from build123d import *

# Parameters (mm, degrees)
F0_W      = 76.2
F0_H      = 76.2
F1_DEPTH  = 76.2
F2_R      = 12.7
F4_DEPTH  = 12.7
F6_DEPTH  = 12.7
F7_W      = 25.4
F7_H      = 25.4
F8_DEPTH  = 25.4
F9_W      = 25.4
F9_H      = 25.4
F10_DEPTH = 25.4
F11_W     = 3.6200266331
F11_H     = 25.4
F12_DEPTH = 12.7
F13_W     = 5.1714666188
F13_H     = 16.2901245058
F13_R     = 2.3271590471
F14_DEPTH = 12.7
F16_DEPTH = 12.7


with BuildPart() as f1:
    # F0 (on Front) → F1 (new body)
    with BuildSketch(Plane.XZ):
        with Locations((38.1, 38.1)):
            Rectangle(F0_W, F0_H)
    extrude(amount=F1_DEPTH)

    # F2
    f2_edges = [f1.edges().sort_by_distance(p)[0] for p in [
        (38.1, -76.2, 76.2),
        (76.2, -38.1, 76.2),
        (38.1, 0, 76.2),
        (0, -38.1, 76.2),
        (76.2, -76.2, 38.1),
        (76.2, 0, 38.1),
        (0, -76.2, 38.1),
        (0, 0, 38.1),
        (0, -38.1, 0),
        (38.1, 0, 0),
        (76.2, -38.1, 0),
        (38.1, -76.2, 0),
    ]]
    fillet(f2_edges, radius=F2_R)

    # F3 (on face) → F4 (cut)
    with BuildSketch(Plane.XZ.offset(76.2)):
        with BuildLine():
            Line((15.24, 47.6933766934), (15.24, 38.1))
            ThreePointArc((15.24, 38.1), (21.992776406, 42.8966883467), (15.24, 47.6933766934))
        make_face()
        Polygon((27.94, 50.8), (27.94, 25.4), (40.64, 25.4), (40.64, 30.5915938972), (34.1505076285, 30.5915938972), (34.1505076285, 35.7831877943), (39.3421015257, 35.7831877943), (39.3421015257, 40.9747816915), (34.1505076285, 40.9747816915), (34.1505076285, 46.1663755887), (40.64, 46.1663755887), (40.64, 50.8), align=None)
        with BuildLine():
            ThreePointArc((45.72, 25.4), (58.42, 38.1), (45.72, 50.8))
            Line((45.72, 50.8), (45.72, 25.4))
        make_face()
    extrude(amount=-F4_DEPTH, mode=Mode.SUBTRACT)

    # F5 (on face) → F6 (cut)
    with BuildSketch(Plane.XZ.offset(76.2)):
        Polygon((23.7294812034, 22.97295762), (15.8522693162, 35.67295762), (15.8522693162, 22.97295762), (18.3922693162, 22.97295762), (18.3922693162, 25.51295762), (21.1894812034, 25.51295762), (21.1894812034, 22.97295762), align=None)
    extrude(amount=-F6_DEPTH, mode=Mode.SUBTRACT)

    # F7 (on face) → F8 (cut)
    with BuildSketch(Plane(origin=(0, 0, 0), x_dir=(1, 0, 0), z_dir=(0, 0, -1))):
        with Locations((38.1038359793, 38.1)):
            Rectangle(F7_W, F7_H)
    extrude(amount=-F8_DEPTH, mode=Mode.SUBTRACT)

    # F9 (on face) → F10 (join)
    with BuildSketch(Plane.XY.offset(76.2)):
        with Locations((38.1, -38.0961640207)):
            Rectangle(F9_W, F9_H)
    extrude(amount=F10_DEPTH)

    # F11 (on face) → F12 (cut)
    with BuildSketch(Plane(origin=(0, 0, 0), x_dir=(0, -1, 0), z_dir=(-1, 0, 0))):
        with BuildLine():
            ThreePointArc((16.548698768, 44.5045307279), (20.8982916063, 50.9688649327), (16.548698768, 57.4331991374))
            Line((16.548698768, 57.4331991374), (16.548698768, 44.5045307279))
        make_face()
        with BuildLine():
            ThreePointArc((16.548698768, 20.9743473679), (23.013450923, 29.5072691515), (16.548698768, 38.0401909351))
            Line((16.548698768, 38.0401909351), (16.548698768, 20.9743473679))
        make_face()
        with Locations((27.4087795988, 32.1229073822)):
            Rectangle(F11_W, F11_H)
        with BuildLine():
            Line((36.9759984314, 37.5230461359), (31.0288090259, 37.5230461359))
            ThreePointArc((31.0288090259, 37.5230461359), (39.5617289469, 24.9625075374), (48.0946488678, 37.5230461359))
            Line((48.0946488678, 37.5230461359), (42.1474650502, 37.5230461359))
            ThreePointArc((42.1474650502, 37.5230461359), (39.5617317408, 29.699298714), (36.9759984314, 37.5230461359))
        make_face()
        Polygon((51.9732572138, 54.6391973982), (51.9732572138, 29.2391973982), (59.5346949809, 30.1820965947), (59.5346949809, 35.2620965947), (53.9881583642, 35.2620965947), (53.9881583642, 40.3420965947), (59.0681583642, 40.3420965947), (59.0681583642, 45.4220965947), (53.9881583642, 45.4220965947), (53.9881583642, 50.5020965947), (58.9798856309, 49.5591973982), (58.9798856309, 54.6391973982), align=None)
    extrude(amount=-F12_DEPTH, mode=Mode.SUBTRACT)

    # F13 (on face) → F14 (cut)
    with BuildSketch(Plane(origin=(0, 0, 0), x_dir=(-1, 0, 0), z_dir=(0, 1, 0))):
        with BuildLine():
            ThreePointArc((-52.724421297, 37.3828077149), (-48.797749492, 44.5476863023), (-56.9577540953, 44.958248733))
            Line((-56.9577540953, 44.958248733), (-56.9577540953, 19.558248733))
            Line((-56.9577540953, 19.558248733), (-52.724421297, 19.558248733))
            Line((-52.724421297, 19.558248733), (-52.724421297, 37.3828077149))
        make_face()
        with Locations((-42.6646117121, 28.6022629589)):
            Rectangle(F13_W, F13_H)
        with BuildLine():
            Line((-37.4931432307, 36.7473252118), (-37.4931432307, 20.7157749683))
            Line((-37.4931432307, 20.7157749683), (-34.9074080586, 20.7157749683))
            Line((-34.9074080586, 20.7157749683), (-34.9074080586, 28.2144043595))
            ThreePointArc((-34.9074080586, 28.2144043595), (-31.9338152185, 31.1879971996), (-28.9602223784, 28.2144043595))
            Line((-28.9602223784, 28.2144043595), (-28.9602223784, 21.2329216301))
            Line((-28.9602223784, 21.2329216301), (-26.4202223784, 21.2329216301))
            Line((-26.4202223784, 21.2329216301), (-27.4545157021, 32.0930033922))
            ThreePointArc((-27.4545157021, 32.0930033922), (-30.6866828045, 35.3251704946), (-33.9188499069, 32.0930033922))
            Line((-33.9188499069, 32.0930033922), (-33.9188499069, 36.7473252118))
            Line((-33.9188499069, 36.7473252118), (-37.4931432307, 36.7473252118))
        make_face()
        Polygon((-23.4643667936, 45.8856336772), (-23.4643667936, 21.2329216301), (-21.2937723845, 21.1951211095), (-21.2937723845, 28.6565385759), (-18.9875140786, 21.1951211095), (-15.4602974653, 21.1951211095), (-21.4294362813, 33.4047153592), (-14.3750030547, 45.6143096089), (-17.0882474631, 45.6143096089), (-21.2937723845, 39.2381884158), (-21.2937723845, 45.8856336772), align=None)
        with Locations((-42.4060374498, 42.69451648)):
            Circle(F13_R)
    extrude(amount=-F14_DEPTH, mode=Mode.SUBTRACT)

    # F15 (on face) → F16 (cut)
    with BuildSketch(Plane.YZ.offset(76.2)):
        with BuildLine():
            Line((-48.0946525931, 37.2644737363), (-53.2661229372, 37.2644737363))
            ThreePointArc((-53.2661229372, 37.2644737363), (-56.8104432824, 35.0391216214), (-56.1766475439, 39.1758717597))
            ThreePointArc((-56.1766475439, 39.1758717597), (-52.9242890713, 42.80015293), (-48.0946525931, 42.1773679554))
            ThreePointArc((-48.0946525931, 42.1773679554), (-55.964214699, 44.1564514691), (-60.2476038039, 37.2644737363))
            ThreePointArc((-60.2476038039, 37.2644737363), (-54.1711281985, 28.6739696125), (-48.0946525931, 37.2644737363))
        make_face()
        with BuildLine():
            Line((-45.0075529516, 37.6416556537), (-45.0075529516, 29.6637304127))
            Line((-45.0075529516, 29.6637304127), (-42.6141768694, 29.6637304127))
            Line((-42.6141768694, 29.6637304127), (-42.2433055937, 34.6854478121))
            ThreePointArc((-42.2433055937, 34.6854478121), (-40.744535625, 36.1842177808), (-39.2457656562, 34.6854478121))
            Line((-39.2457656562, 34.6854478121), (-39.2457656562, 36.2912714481))
            ThreePointArc((-39.2457656562, 36.2912714481), (-40.744535625, 37.7900414169), (-42.2433055937, 36.2912714481))
            Line((-42.2433055937, 36.2912714481), (-42.2433055937, 37.6416556537))
            Line((-42.2433055937, 37.6416556537), (-45.0075529516, 37.6416556537))
        make_face()
        with BuildLine():
            ThreePointArc((-31.9660305977, 33.0967174506), (-31.3338769664, 34.1906255239), (-31.1143183532, 35.4348309338))
            ThreePointArc((-31.1143183532, 35.4348309338), (-31.3338769664, 36.6790363437), (-31.9660305977, 37.772944417))
            Line((-31.9660305977, 37.772944417), (-31.9660305977, 33.0967174506))
        make_face()
        with BuildLine():
            ThreePointArc((-31.9660305977, 37.772944417), (-31.3338769664, 36.6790363437), (-31.1143183532, 35.4348309338))
            ThreePointArc((-31.1143183532, 35.4348309338), (-31.3338769664, 34.1906255239), (-31.9660305977, 33.0967174506))
            Line((-31.9660305977, 33.0967174506), (-31.9660305977, 31.4737968147))
            Line((-31.9660305977, 31.4737968147), (-29.7178756446, 31.4737968147))
            Line((-29.7178756446, 31.4737968147), (-29.7178756446, 39.5029187202))
            Line((-29.7178756446, 39.5029187202), (-31.9660305977, 39.5029187202))
            Line((-31.9660305977, 39.5029187202), (-31.9660305977, 37.772944417))
        make_face()
        with BuildLine():
            Line((-31.9660305977, 33.0967174506), (-31.9660305977, 37.772944417))
            ThreePointArc((-31.9660305977, 37.772944417), (-38.3846005973, 35.4348309338), (-31.9660305977, 33.0967174506))
        make_face()
        Polygon((-24.1510178894, 41.751075536), (-27.0415022969, 41.751075536), (-22.9996046927, 31.2696424589), (-26.7875780846, 21.3012932532), (-24.2580734193, 20.3400813043), (-16.1218941212, 41.751075536), (-19.5476543158, 41.751075536), (-22.6522479206, 34.0431183577), align=None)
    extrude(amount=-F16_DEPTH, mode=Mode.SUBTRACT)


solid = f1.part
Work out the finished part from the listing and answer in its coordinate system (mm). A direction names the side the tool comes from. Coordinates: 2 decimals unless noted, no trailing zeros. Loops run counter-clockwise (first coordinate to the right, second up) from the corner with the lowest first, then second, coordinate; pieces in that order, holes last. Notation, with made-up numbers: (-2, 47) -> (57, 47) arc R20 ccw to (57, 61) -> close; hole circle Ø6 at (11, 89). An arc over 180 degrees is marked (long way). Write each question's results on one line, items separated by ' | '. Start each with the question number.
1) Consider line 1 along Z through (x, y) = (5.5, -36); line 2 along Y through (x, z) = (41.5, 18); line 3 along Z through (x, y) = (64.5, -55). Determine where each line is inside the solid, lowest interval first.
2) For faces 5 (the cylindrical face through (30.616, -6.261, 35.324)), 6 (the flat face through (18, -63.5, 43)), 7 (the flat face through (6, -27, 19.423)), determine the directions among +Z, -Z, +X, -X, +Y, -Y from which every point of the face is accessible in a straight line to the end or side of a thin tool.
3) Find section D-D on x = 47. Determine the outline of the cut face in (y, z).
4) The mould has two halves that part along Y. Classify faces 1 (the cylindrical face through (3.62, -72.38, 38.46)), 2 (the flat face through (17.952, -6.261, 39.424)), 3 (the flat face through (50.804, -38, 13)), 4 (the flat face through (38, 0, 38)): pulls with the +Y half, pulls with the -Y half, needs draft (parallel to the pull), parting line crosses it, or undercut.
5) Find section B-B on z = 62. Determine the outline of the cut face in (x, y), then the cut area to 3 significant figures.
6) Flat-ended cylindrical pins translate along their axes: P1, Ø2.5, axis at x = 69.5, z = 36, coming from the -Y side; P2, Ø2.5, axis at x = 4.5, z = 32, coming from the +Y side; P3, Ø5.5, axis at x = 67, y = -50, coming from the -Z side. Find the tip coordinate at first contact, or state that the pin passes through.
7) Find section A-A on x = 10. Count the separate pieces of the cut face and the enclosed holes in it, then the cut area to 3 significant figures.
Response values:
1) line 1: z = 2.24 to 25.68, 31.56 to 36.52, 37.52 to 73.96 | line 2: y = -76.2 to -50.8, -25.4 to 0 | line 3: z = 0.04 to 28.73, 34.73 to 41.39, 44.47 to 76.16
2) face 5: +Y | face 6: -Y | face 7: -X
3) outline: (-76.2, 12.7) arc R12.7 ccw to (-63.5, 0) -> (-50.8, 0) -> (-50.8, 25.4) -> (-25.4, 25.4) -> (-25.4, 0) -> (-12.7, 0) arc R12.7 ccw to (0, 12.7) -> (0, 63.5) arc R12.7 ccw to (-12.7, 76.2) -> (-25.4, 76.2) -> (-25.4, 101.6) -> (-50.8, 101.6) -> (-50.8, 76.2) -> (-63.5, 76.2) arc R12.7 ccw to (-76.2, 63.5) -> (-76.2, 50.74) -> (-63.5, 50.74) -> (-63.5, 25.46) -> (-76.2, 25.46) -> close
4) face 1: pulls with the -Y half | face 2: needs draft | face 3: undercut | face 4: pulls with the +Y half
5) outline: (0, -63.5) arc R12.7 ccw to (12.7, -76.2) -> (63.5, -76.2) arc R12.7 ccw to (76.2, -63.5) -> (76.2, -12.7) arc R12.7 ccw to (63.5, 0) -> (12.7, 0) arc R12.7 ccw to (0, -12.7) -> close | area: 5,670 mm^2
6) P1: stops at y = -75.28 | P2: stops at y = -2.07 | P3: stops at z = 0.02
7) separate pieces: 1 | enclosed holes: 5 | area: 5,110 mm^2
